Geometry check sheet. Reference: the model listing, model coordinates, mm. A direction names the side the tool comes from. Give positions to 0.01 mm unless a question says otherwise; leave off trailing zeros. Write each loop counter-clockwise with the first axis right and the second up, starting at its lowest first coordinate (ties: lowest second). Pieces come first, ordered by that corner, then holes. Notation, with made-up numbers: M -27,-33.75 L -13,-33.75 A28 cw -13,-5.75 Z; hole C -19.75,8.25 d3. An arc over 180 degrees is marked long. Use one line per item in the form item = value. Start each with the question number.
```python
from build123d import *

# Parameters (mm, degrees)
SKETCH_1_W               = 26
SKETCH_1_H               = 11
SKETCH_1_R               = 1
EXTRUDE_1_DEPTH          = 2
SKETCH_2_R               = 3.315
EXTRUDE_2_DEPTH          = 26
FILLET_1_R               = 10
CUT_EXTRUDE_1_DEPTH      = 18.748239349
CUT_EXTRUDE_1_DEPTH_BACK = 18.748239349
SKETCH_3_W               = 10
SKETCH_3_H               = 7


with BuildPart() as part:
    # 草图1 → 凸台-拉伸1 (new body)
    with BuildSketch(Plane(origin=(0, 0, 0), x_dir=(1, 0, 0), z_dir=(0, 1, 0))):
        with Locations((0, -5.5)):
            Rectangle(SKETCH_1_W, SKETCH_1_H)
        with Locations(Location((9, -7.5, 0), (0, 0, 270))):
            Circle(SKETCH_1_R, mode=Mode.SUBTRACT)
        with Locations(Location((-9, -7.5, 0), (0, 0, 90))):
            Circle(SKETCH_1_R, mode=Mode.SUBTRACT)
    extrude(amount=EXTRUDE_1_DEPTH)

    # 草图2 → 凸台-拉伸2 (add)
    with BuildSketch(Plane(origin=(13, 0, 0), x_dir=(0, 0, -1), z_dir=(1, 0, 0))):
        with Locations((0, 3.685)):
            Circle(SKETCH_2_R)
    extrude(amount=-EXTRUDE_2_DEPTH)

    # 圆角1
    # the kernel refuses this fillet: 10 mm, written as the material it takes off along each edge
    with BuildSketch(Plane(origin=(19.737534787, 0, 0), x_dir=(0, 1, 0), z_dir=(-1, 0, 0))) as fillet_1_piece_1:
        with BuildLine():
            CenterArc((10, -2.695013915), FILLET_1_R, 164.365401099, 15.634598901)
            Line((0, -2.695013915), (-0.2, -2.695013915))
            Line((-0.2, -2.695013915), (-0.2, 0))
            Line((-0.2, 0), (0, 0.2))
            ThreePointArc((0, 0.2), (0.185, 0.2), (0.1774, 0.053900278))
            Line((0.1774, 0.053900278), (0.37, 0))
        make_face()
    extrude(amount=39.475069573, mode=Mode.SUBTRACT)

    # 草图3 → 切除-拉伸1 (cut, two sides: drawn at the far end of the back side and taken through both)
    with BuildSketch(Plane(origin=(0, 2, 0), x_dir=(1, 0, 0), z_dir=(0, 1, 0)).offset(-CUT_EXTRUDE_1_DEPTH_BACK)):
        with Locations((0, 0.185)):
            Rectangle(SKETCH_3_W, SKETCH_3_H)
    extrude(amount=CUT_EXTRUDE_1_DEPTH + CUT_EXTRUDE_1_DEPTH_BACK, mode=Mode.SUBTRACT)


solid = part.part
```
(1) Tool access check on faces 1 (the flat face through (-5, 3, 0)), 2 (the flat face through (0, 1, 11)). Record the directions out of +Z, -Z, +X, -X, +Y, -Y that give a thin tool (end or side, any length) a straight path to the whole face; none if there is none.
(2) Sectioned sample at B-B, the plane y = 6.5. Record the boundary of the cut face in (x, z), plus the area to 3 significant figures.
(3) Draft check along X on faces 3 (the cylindrical face through (-9.99, 0.99, 7.63)), 4 (the cylindrical face through (-8.94, 6.5, -1.75)), 5 (the flat face through (-13, 3, 2)). Enter one of: released by +X, released by -X, zero draft, split by the parting line, or undercut.
(4) Sectioned sample at A-A, the plane z = 7.5. Record the boundary of the cut face in (x, y), plus the area to 3 significant figures.
(5) Thickness scan on probe 1 along X at (y, z) = (1.6, 7.5); probe 2 along X at (y, z) = (1, 3); probe 3 along Z at (x, y) = (-11.5, 3.5). Record the ranges inside material, lowest first. Write a range as [from, to].
(6) Sectioned sample at D-D, the plane y = 1.5. Record the boundary of the cut face in (x, z) (3 decimals).
(7) Depth check by flat-ended pin: pin 1 (2.5 mm diameter, centred on x = -9, z = 7.5, fed in from +Y); pin 2 (2 mm diameter, centred on x = 2, y = 1, fed in from -Z) (3 decimals); pin 3 (5 mm diameter, centred on x = -3, z = 0, fed in from -Y). Enter the tip coordinate at first touch or a pass-through.
(8) Sectioned sample at C-C, the plane x = 9. Record the boundary of the cut face in (y, z) (3 decimals), plus the area to 3 significant figures.
Numbers:
q1.face_1 = -Z, +Y, -Y
q1.face_2 = +Z, +X, -X, +Y, -Y
q2.outline = M -13,-1.75 L -5,-1.75 L -5,1.75 L -13,1.75 Z; M 5,-1.75 L 13,-1.75 L 13,1.75 L 5,1.75 Z
q2.area = 56.0 mm2
q3.face_3 = undercut
q3.face_4 = zero draft
q3.face_5 = released by -X
q4.outline = M -13,0 L -10,0 L -10,2 L -13,2 Z; M -8,0 L 8,0 L 8,2 L -8,2 Z; M 10,0 L 13,0 L 13,2 L 10,2 Z
q4.area = 44.0 mm2
q5.probe_1 = [-13, -10], [-8, 8], [10, 13]
q5.probe_2 = [-13, -5], [5, 13]
q5.probe_3 = [-3.31, 3.31]
q6.outline = M -13,-2.493 L -5,-2.493 L -5,3.315 L 5,3.315 L 5,-2.493 L 13,-2.493 L 13,11 L -13,11 Z; hole C -9,7.5 d2; hole C 9,7.5 d2
q7.pin_1 = 2
q7.pin_2 = 3.315
q7.pin_3 = 0.07
q8.outline = M 0,2.695 A10 ccw 0.37,0 A3.315 ccw long 2,2.855 L 2,6.5 L 0,6.5 Z; M 0,8.5 L 2,8.5 L 2,11 L 0,11 Z
q8.area = 48.9 mm2
